Verification items for the finished model (mm, model axes). A direction names the side the tool comes from. Give positions to 0.01 mm unless a question says otherwise; leave off trailing zeros. Write each loop counter-clockwise with the first axis right and the second up, starting at its lowest first coordinate (ties: lowest second). Pieces come first, ordered by that corner, then holes. Notation, with made-up numbers: (-19, -23) - (38, -23) arc R11 ccw to (38, -10) - close; hole circle Ø10 at (63.5, -3.5). An arc over 180 degrees is marked (long way). Put each result on its own line as item: value.
from build123d import *

# Parameters (mm, degrees)
BOSS_EXTRUDE1_DEPTH      = 40
BOSS_EXTRUDE1_DEPTH_BACK = 7
SKETCH1_R                = 1.5
CHAMFER1_SIZE            = 0.5
CUT_EXTRUDE1_DEPTH       = 1
CUT_EXTRUDE1_DEPTH_BACK  = 1
SKETCH2_R                = 1


with BuildPart() as part:
    # Sketch1 → Boss-Extrude1 (new, two sides: drawn at the far end of the back side and taken through both)
    with BuildSketch(Plane.XY.offset(-BOSS_EXTRUDE1_DEPTH_BACK)):
        Circle(SKETCH1_R)
    extrude(amount=BOSS_EXTRUDE1_DEPTH + BOSS_EXTRUDE1_DEPTH_BACK)

    # Chamfer1
    chamfer1_edges = [part.edges().sort_by_distance(p)[0] for p in [
        (-1.5, 0, 40),
        (-1.5, 0, -7),
    ]]
    chamfer(chamfer1_edges, length=CHAMFER1_SIZE)

    # Sketch2 → Cut-Extrude1 (cut, two sides: drawn at the far end of the back side and taken through both)
    with BuildSketch(Plane.XY.offset(16.5).offset(-CUT_EXTRUDE1_DEPTH_BACK)):
        Circle(SKETCH2_R)
    extrude(amount=CUT_EXTRUDE1_DEPTH + CUT_EXTRUDE1_DEPTH_BACK, mode=Mode.SUBTRACT)


solid = part.part
Q1. Release check for a two-part mould opening along X. For faces 3 (the face through (0, 0, 40)), 4 (the face through (-1.5, 0.07, 16.18)), 5 (the face through (0, -1, 16)) record: released by +X, released by -X, zero draft, split by the parting line, or undercut.
Answers follow:
face 3: zero draft
face 4: split by the parting line
face 5: undercut
Q2. Scan lines: line 1 along Z through (x, y) = (0.9, -0.35); line 2 along Y through (x, z) = (0, 16.8); line 3 along Y through (x, z) = (0.1, 9.5). Record each from-to range of solid material in increasing order.
Answers follow:
line 1: z = -7 to 15.5, 17.5 to 40
line 2: y = -1.5 to -1, 1 to 1.5
line 3: y = -1.5 to 1.5
Q3. Section check D-D, the plane z = 9.5. Record the cut outline in (x, y).
Answers follow:
outline: circle Ø3 at (0, 0)
Q4. Section check A-A, the plane x = 0. Record the cut outline in (y, z).
Answers follow:
outline: (-1.5, -6.5) - (-1, -7) - (1, -7) - (1.5, -6.5) - (1.5, 39.5) - (1, 40) - (-1, 40) - (-1.5, 39.5) - close; hole (-1, 15.5) - (1, 15.5) - (1, 17.5) - (-1, 17.5) - close
Q5. Section check C-C, the plane z = 16. Record the cut outline in (x, y).
Answers follow:
outline: circle Ø3 at (0, 0); hole circle Ø2 at (0, 0)
Q6. Set-up check for faces 1 (the face through (0, 0, -7)), 2 (the face through (0, 0, 15.5)): record each of +Z, -Z, +X, -X, +Y, -Y from which the full face is reachable in a straight line by a thin tool's end or side.
Answers follow:
face 1: -Z, +X, -X, +Y, -Y
face 2: none
